```python
from build123d import *

# Parameters (mm, degrees)
SKETCH2_R           = 22.5
BOSS_EXTRUDE1_DEPTH = 118.8
SKETCH3_R           = 11.25
CUT_EXTRUDE1_DEPTH  = 35
SKETCH4_W           = 6
SKETCH4_H           = 6
CUT_EXTRUDE2_DEPTH  = 35
SKETCH5_R           = 21
CUT_EXTRUDE3_DEPTH  = 25
BOSS_EXTRUDE2_START = -118.8
SKETCH6_R           = 22.5
BOSS_EXTRUDE2_DEPTH = 118.8


with BuildPart() as part:
    # Sketch2 → Boss-Extrude1 (new body)
    with BuildSketch(Plane.XY):
        Circle(SKETCH2_R)
    extrude(amount=BOSS_EXTRUDE1_DEPTH)

    # Sketch3 → Cut-Extrude1 (cut)
    with BuildSketch(Plane(origin=(0, 0, 0), x_dir=(-1, 0, 0), z_dir=(0, 0, -1))):
        Circle(SKETCH3_R)
    extrude(amount=-CUT_EXTRUDE1_DEPTH, mode=Mode.SUBTRACT)

    # Sketch4 → Cut-Extrude2 (cut)
    with BuildSketch(Plane(origin=(0, 0, 0), x_dir=(-1, 0, 0), z_dir=(0, 0, -1))):
        with Locations((0, 13.842624221)):
            Rectangle(SKETCH4_W, SKETCH4_H)
    extrude(amount=-CUT_EXTRUDE2_DEPTH, mode=Mode.SUBTRACT)

    # Sketch5 → Cut-Extrude3 (cut)
    with BuildSketch(Plane.XY.offset(118.8)):
        Circle(SKETCH5_R)
    extrude(amount=-CUT_EXTRUDE3_DEPTH, mode=Mode.SUBTRACT)

    # Sketch6 → Boss-Extrude2 (add)
    with BuildSketch(Plane.XY.offset(118.8).offset(BOSS_EXTRUDE2_START)):
        Polygon((-4.44294699, 23.55705301), (0, 28), (4.44294699, 23.55705301), (10.252068727, 21.66955494), (16.457987064, 22.652475842), (17.440907967, 16.446557506), (21.031142645, 11.505023404), (26.629582456, 8.652475842), (23.777034895, 3.054036032), (23.777034895, -3.054036032), (26.629582456, -8.652475842), (21.031142645, -11.505023404), (17.440907967, -16.446557506), (16.457987064, -22.652475842), (10.252068727, -21.66955494), (4.44294699, -23.55705301), (0, -28), (-4.44294699, -23.55705301), (-10.252068727, -21.66955494), (-16.457987064, -22.652475842), (-17.440907967, -16.446557506), (-21.031142645, -11.505023404), (-26.629582456, -8.652475842), (-23.777034895, -3.054036032), (-23.777034895, 3.054036032), (-26.629582456, 8.652475842), (-21.031142645, 11.505023404), (-17.440907967, 16.446557506), (-16.457987064, 22.652475842), (-10.252068727, 21.66955494), align=None)
        Circle(SKETCH6_R, mode=Mode.SUBTRACT)
    extrude(amount=BOSS_EXTRUDE2_DEPTH)


solid = part.part
```
Geometry: final body of the model. Coordinates: model frame, mm. A direction names the side the tool comes from. Give positions to 0.01 mm unless a question says otherwise; leave off trailing zeros. Order: outer loops, then holes, each group sorted by start corner. A loop starts at its lowest first (then second) coordinate and runs counter-clockwise, first axis right, second up. Notation, with made-up numbers: (88.25, 42) -> (97.25, 42) arc R16 ccw to (97.25, 61) -> close; hole circle Ø2 at (-2.75, -20). An arc over 180 degrees is marked (long way). Write each question's results on one line, items separated by ' | '. Start each with the question number.
1) Section B-B (y = 0). Return loops of the section in (x, z), then the cut area to 3 significant figures.
2) First-contact query: pin 1 (7 mm diameter, centred on x = 2, y = 7, fed in from -Z); pin 2 (3 mm diameter, centred on x = 20.5, z = 63.5, fed in from -Y); pin 3 (5 mm diameter, centred on y = -14.5, z = 58, fed in from -X). Flat tips, straight axial feed; report the tip coordinate or a pass-through.
3) Line query: line 1 (Y direction, x = 0, z = 11); line 2 (Y direction, x = 0, z = 113); line 3 (X direction, y = 0, z = 20). Output: solid intervals per line, ascending. Write a range as from..to.
4) Draft query along X for faces 1 (the flat face through (19.26, -13.94, 58.57)), 2 (the flat face through (-16.956, 19.506, 58.568)), 3 (the flat face through (4, -21, 118.8)), 4 (the flat face through (13.312, 22.154, 58.568)). Return one class per face: pulls with the +X half, pulls with the -X half, needs draft (parallel to the pull), parting line crosses it, or undercut.
5) Set-up query: faces 5 (the flat face through (-7.39, 22.6, 58.57)), 6 (the cylindrical face through (20.03, 6.31, 106.48)), 7 (the flat face through (-13.312, -22.154, 58.568)), 8 (the flat face through (-23.777, 0, 59)), 9 (the cylindrical face through (0.45, -11.24, 17.26)). Return all of +Z, -Z, +X, -X, +Y, -Y with unobstructed straight access to the full face (end or side cutting, diameter ignored); none if empty.
6) Section C-C (x = -14). Return loops of the section in (y, z).
Calculated:
1) outline: (-23.78, 0) -> (-11.25, 0) -> (-11.25, 35) -> (11.25, 35) -> (11.25, 0) -> (23.78, 0) -> (23.78, 118.8) -> (21, 118.8) -> (21, 93.8) -> (-21, 93.8) -> (-21, 118.8) -> (-23.78, 118.8) -> close | area: 3,810 mm2
2) pin 1: z = 35 | pin 2: y = -14.3 | pin 3: x = -20.67
3) line 1: -28..-11.25, 16.84..28 | line 2: -28..-21, 21..28 | line 3: -23.78..-11.25, 11.25..23.78
4) face 1: pulls with the +X half | face 2: pulls with the -X half | face 3: needs draft | face 4: undercut
5) face 5: +Z, -Z, +Y | face 6: +Z | face 7: +Z, -Z, -Y | face 8: +Z, -Z, -X | face 9: -Z
6) outline: (-22.26, 0) -> (22.26, 0) -> (22.26, 118.8) -> (15.65, 118.8) -> (15.65, 93.8) -> (-15.65, 93.8) -> (-15.65, 118.8) -> (-22.26, 118.8) -> close
